CAD build for the part. Positions are in the model's coordinates, mm. A direction names the side the tool comes from. Round coordinates to 2 decimals unless told otherwise and drop trailing zeros. Loops run counter-clockwise (first coordinate to the right, second up) from the corner with the lowest first, then second, coordinate; pieces in that order, holes last. Notation, with made-up numbers: (62.25, 7.5) - (105.25, 7.5) arc R5 ccw to (105.25, 13.5) - close; hole circle Ø5 at (18.25, 2.25). An arc over 180 degrees is marked (long way). Use one line per item in the form item = value.
from build123d import *

# Parameters (mm, degrees)
F0_R     = 1.4
F1_DEPTH = 15
F2_W     = 5.37
F2_H     = 2.4
F3_DEPTH = 9.3


with BuildPart() as f1:
    # F0 (on Top) → F1 (new body)
    with BuildSketch(Plane.XY):
        with BuildLine():
            Line((-1.65, 5.35), (-1.65, 6.9570108524))
            ThreePointArc((-1.65, 6.9570108524), (-7.15, 0), (-1.65, -6.9570108524))
            Line((-1.65, -6.9570108524), (-1.65, -5.35))
            Line((-1.65, -5.35), (-1.65, 5.35))
        make_face()
        with BuildLine():
            Line((5.15, -4.9598387071), (5.15, 4.9598387071))
            ThreePointArc((5.15, 4.9598387071), (4.9505533954, 5.1589263494), (4.7434164903, 5.35))
            Line((4.7434164903, 5.35), (-1.65, 5.35))
            Line((-1.65, 5.35), (-1.65, -5.35))
            Line((-1.65, -5.35), (4.7434164903, -5.35))
            ThreePointArc((4.7434164903, -5.35), (4.9505533954, -5.1589263494), (5.15, -4.9598387071))
        make_face()
        Circle(F0_R, mode=Mode.SUBTRACT)
    extrude(amount=F1_DEPTH)

    # F2 (on face) → F3 (cut)
    with BuildSketch(Plane.YZ.offset(5.15)):
        with Locations((0, 7)):
            Rectangle(F2_W, F2_H)
    extrude(amount=-F3_DEPTH, mode=Mode.SUBTRACT)


solid = f1.part
1) Two-plate mould, pull along Z, no slides. Class faces 4 (the flat face through (-4.15, 0, 7)), 5 (the flat face through (1, 2.685, 7)), 6 (the flat face through (5.15, 0, 9)), 7 (the flat face through (-1, 2, 15)): +Z half, -Z half, draft (parallel to the pull), parting line (faces both ways), or undercut.
Report:
face_4 = undercut
face_5 = undercut
face_6 = draft
face_7 = +Z half
2) Tool access for faces 1 (the flat face through (2, -5.35, 7)), 2 (the flat face through (-1.65, 6, 7)), 3 (the flat face through (2, 0, 8.2)): list every direction of +Z, -Z, +X, -X, +Y, -Y with a clear straight run to the whole face (end or side of a thin tool).
Report:
face_1 = +Z, -Z, +X, -Y
face_2 = +Z, -Z, +X, +Y
face_3 = +X
3) Slice it at C-C (z = 10.5). Write the cut outline in (x, y).
Report:
outline = (-1.65, -6.96) - (-1.65, -5.35) - (4.74, -5.35) arc R7.15 ccw to (5.15, -4.96) - (5.15, 4.96) arc R7.15 ccw to (4.74, 5.35) - (-1.65, 5.35) - (-1.65, 6.96) arc R7.15 ccw to start; hole circle Ø2.8 at (0, 0)
4) Slice it at D-D (x = 0). Write the cut outline in (y, z) (3 decimals).
Report:
outline = (-5.35, 0) - (-1.4, 0) - (-1.4, 5.8) - (-2.685, 5.8) - (-2.685, 8.2) - (-1.4, 8.2) - (-1.4, 15) - (-5.35, 15) - close; (1.4, 0) - (5.35, 0) - (5.35, 15) - (1.4, 15) - (1.4, 8.2) - (2.685, 8.2) - (2.685, 5.8) - (1.4, 5.8) - close
5) Slice it at B-B (y = 0). Write the cut outline in (x, z).
Report:
outline = (-7.15, 0) - (-1.4, 0) - (-1.4, 5.8) - (-4.15, 5.8) - (-4.15, 8.2) - (-1.4, 8.2) - (-1.4, 15) - (-7.15, 15) - close; (1.4, 0) - (5.15, 0) - (5.15, 5.8) - (1.4, 5.8) - close; (1.4, 8.2) - (5.15, 8.2) - (5.15, 15) - (1.4, 15) - close
6) Drill centre lines: probe 1 along Z at (x, y) = (-3.25, 1); probe 2 along Y at (x, z) = (0, 3.65); probe 3 along X at (y, z) = (0, 2.95). Where is each one in solid material? Low to high.
Report:
probe_1 = 0 to 5.8, 8.2 to 15
probe_2 = -5.35 to -1.4, 1.4 to 5.35
probe_3 = -7.15 to -1.4, 1.4 to 5.15
7) Slice it at A-A (x = 3). Write the cut outline in (y, z) (3 decimals).
Report:
outline = (-5.35, 0) - (5.35, 0) - (5.35, 15) - (-5.35, 15) - close; hole (-2.685, 5.8) - (2.685, 5.8) - (2.685, 8.2) - (-2.685, 8.2) - close
8) Flat gauge pins, fed straight in: pin 1 (1.5 mm diameter, centred on x = -3.5, z = 7.5, fed in from -Y); pin 2 (5 mm diameter, centred on x = 3.5, z = 7.5, fed in from +Y); pin 3 (2 mm diameter, centred on y = 1.5, z = 13, fed in from -X). Where does each tip first touch, or does it go through?
Report:
pin_1 = -6.6
pin_2 = 5.35
pin_3 = -7.13
